Input: part model. Units: mm. Frame: model coordinates. A direction names the side the tool comes from. Round coordinates to 2 decimals unless told otherwise and drop trailing zeros. Loops run counter-clockwise (first coordinate to the right, second up) from the corner with the lowest first, then second, coordinate; pieces in that order, holes last. Notation, with made-up numbers: (44.5, -11) -> (69.5, -11) arc R20 cw to (69.5, -3) -> close; hole circle Ø5 at (31, 22). An arc over 180 degrees is marked (long way). Answer as a JSON object with one key per item and string values.
```python
from build123d import *

# Parameters (mm, degrees)
SKETCH1_R           = 1.25
BOSS_EXTRUDE1_DEPTH = 10


with BuildPart() as part:
    # Sketch1 → Boss-Extrude1 (new body)
    with BuildSketch(Plane.XY):
        with BuildLine():
            Line((-3.25, 0), (-3.25, -60))
            ThreePointArc((-3.25, -60), (-1.580508653, -64.030508653), (2.45, -65.7))
            Line((2.45, -65.7), (7.45, -65.7))
            Line((7.45, -65.7), (7.45, -62.7))
            Line((7.45, -62.7), (2.45, -62.7))
            ThreePointArc((2.45, -62.7), (0.540811691, -61.909188309), (-0.25, -60))
            Line((-0.25, -60), (-0.25, -3.240370349))
            ThreePointArc((-0.25, -3.240370349), (2.384848004, 2.207940217), (-3.25, 0))
        make_face()
        Circle(SKETCH1_R, mode=Mode.SUBTRACT)
    extrude(amount=BOSS_EXTRUDE1_DEPTH)


solid = part.part
```
1) Reachability of faces 1 (the face through (2.458, 2.127, 4.93)), 2 (the face through (0.56, -61.93, 4.93)) from +Z, -Z, +X, -X, +Y, -Y: full face, straight path, thin tool, end or side. Return the list, or none.
Output:
{"face 1": "+Z, -Z", "face 2": "+Z, -Z, +X"}
2) Section B-B, the plane y = -11.5. Output: boundary loops of the cut face in (x, z), plus the area to 3 significant figures.
Output:
{"outline": "(-3.25, 0) -> (-0.25, 0) -> (-0.25, 10) -> (-3.25, 10) -> close", "area": "30.0 mm^2"}
3) Section C-C, the plane x = 6.75. Output: boundary loops of the cut face in (y, z), plus the area to 3 significant figures.
Output:
{"outline": "(-65.7, 0) -> (-62.7, 0) -> (-62.7, 10) -> (-65.7, 10) -> close", "area": "30.0 mm^2"}
4) Contact query for flat-ended pins moving along their axis: P1, Ø2.5, axis at x = 5.5, z = 7.5, coming from the +Y side; P2, Ø1.5, axis at x = -0.5, z = 5, coming from the -Y side; P3, Ø3, axis at y = -20, z = 4.5, coming from the +X side. Output: stop coordinate, or through.
Output:
{"P1": "stops at y = -62.7", "P2": "stops at y = -65.26", "P3": "stops at x = -0.25"}
5) Ray query, probe 1 along Y at (x, z) = (0, 5); probe 2 along Y at (x, z) = (3.75, 3.5); probe 3 along Y at (x, z) = (-0.75, 7.5). Return the intervals inside material, ascending.
Output:
{"probe 1": "y = -65.15 to -61.13, -3.25 to -1.25, 1.25 to 3.25", "probe 2": "y = -65.7 to -62.7", "probe 3": "y = -64.72 to -1, 1 to 3.16"}
6) Section A-A, the plane z = 5. Output: boundary loops of the cut face in (x, y), plus the area to 3 significant figures.
Output:
{"outline": "(-3.25, -60) arc R5.7 ccw to (2.45, -65.7) -> (7.45, -65.7) -> (7.45, -62.7) -> (2.45, -62.7) arc R2.7 cw to (-0.25, -60) -> (-0.25, -3.24) arc R3.25 ccw (long way) to (-3.25, 0) -> close; hole circle Ø2.5 at (0, 0)", "area": "236 mm^2"}
